```python
from build123d import *

# Parameters (mm, degrees)
SKETCH1_W          = 82.5
SKETCH1_H          = 56
MAINSHAPE_DEPTH    = 4.5
SKETCH2_W          = 10
SKETCH2_H          = 9
TAB1_DEPTH         = 4.5
CUT_EXTRUDE2_DEPTH = 53.707328712
SKETCH5_R          = 1.6
SKETCH5_W          = 4.7
SKETCH5_H          = 10.2
CUT_EXTRUDE3_DEPTH = 53.707328712
SKETCH6_R          = 11.5
CUT_EXTRUDE4_DEPTH = 53.707328712
SKETCH8_R          = 1.6
CUT_EXTRUDE6_DEPTH = 53.707328712
CUT_EXTRUDE7_DEPTH = 53.707328712


with BuildPart() as part:
    # Sketch1 → MainShape (new body)
    with BuildSketch(Plane(origin=(0, 0, 0), x_dir=(1, 0, 0), z_dir=(0, 1, 0))):
        Rectangle(SKETCH1_W, SKETCH1_H)
    extrude(amount=MAINSHAPE_DEPTH)

    # Sketch2 → Tab1 (add, through all)
    with BuildSketch(Plane(origin=(0, 4.5, 0), x_dir=(1, 0, 0), z_dir=(0, 1, 0))):
        with Locations((0, 28)):
            Rectangle(SKETCH2_W, SKETCH2_H)
    extrude(amount=-TAB1_DEPTH)

    # Sketch4 → Cut-Extrude2 (cut, through all)
    with BuildSketch(Plane(origin=(0, 4.5, 0), x_dir=(1, 0, 0), z_dir=(0, 1, 0))):
        with BuildLine():
            Line((-28.25, 17.5), (-31.75, 17.5))
            Line((-31.75, 17.5), (-31.75, 20))
            Line((-31.75, 20), (-32.75, 20))
            ThreePointArc((-32.75, 20), (-32.926776695, 20.073223305), (-33, 20.25))
            Line((-33, 20.25), (-33, 23.95))
            ThreePointArc((-33, 23.95), (-32.926776695, 24.126776695), (-32.75, 24.2))
            Line((-32.75, 24.2), (-31.75, 24.2))
            Line((-31.75, 24.2), (-31.75, 28))
            Line((-31.75, 28), (-28.25, 28))
            Line((-28.25, 28), (-28.25, 24.2))
            Line((-28.25, 24.2), (-27.25, 24.2))
            ThreePointArc((-27.25, 24.2), (-27.073223305, 24.126776695), (-27, 23.95))
            Line((-27, 23.95), (-27, 20.25))
            ThreePointArc((-27, 20.25), (-27.073223305, 20.073223305), (-27.25, 20))
            Line((-27.25, 20), (-28.25, 20))
            Line((-28.25, 20), (-28.25, 17.5))
        make_face()
        with BuildLine():
            Line((28.25, 17.5), (28.25, 20))
            Line((28.25, 20), (27.25, 20))
            ThreePointArc((27.25, 20), (27.073223305, 20.073223305), (27, 20.25))
            Line((27, 20.25), (27, 23.95))
            ThreePointArc((27, 23.95), (27.073223305, 24.126776695), (27.25, 24.2))
            Line((27.25, 24.2), (28.25, 24.2))
            Line((28.25, 24.2), (28.25, 28))
            Line((28.25, 28), (31.75, 28))
            Line((31.75, 28), (31.75, 24.2))
            Line((31.75, 24.2), (32.75, 24.2))
            ThreePointArc((32.75, 24.2), (32.926776695, 24.126776695), (33, 23.95))
            Line((33, 23.95), (33, 20.25))
            ThreePointArc((33, 20.25), (32.926776695, 20.073223305), (32.75, 20))
            Line((32.75, 20), (31.75, 20))
            Line((31.75, 20), (31.75, 17.5))
            Line((31.75, 17.5), (28.25, 17.5))
        make_face()
    extrude(amount=-CUT_EXTRUDE2_DEPTH, mode=Mode.SUBTRACT)

    # Sketch5 → Cut-Extrude3 (cut, through all)
    with BuildSketch(Plane(origin=(0, 4.5, 0), x_dir=(1, 0, 0), z_dir=(0, 1, 0))):
        with Locations(Location((34.5, -4.5, 0), (0, 0, 270))):
            Circle(SKETCH5_R)
        with Locations(Location((-34.5, -4.5, 0), (0, 0, 90))):
            Circle(SKETCH5_R)
        with Locations((34.5, 8)):
            Rectangle(SKETCH5_W, SKETCH5_H)
        with Locations((-34.5, 8)):
            Rectangle(SKETCH5_W, SKETCH5_H)
        with Locations((-34.5, -17)):
            Rectangle(SKETCH5_W, SKETCH5_H)
        with Locations((34.5, -17)):
            Rectangle(SKETCH5_W, SKETCH5_H)
    extrude(amount=-CUT_EXTRUDE3_DEPTH, mode=Mode.SUBTRACT)

    # Sketch6 → Cut-Extrude4 (cut, through all)
    with BuildSketch(Plane(origin=(0, 4.5, 0), x_dir=(1, 0, 0), z_dir=(0, 1, 0))):
        with Locations(Location((-13, 2, 0), (0, 0, 270))):
            Circle(SKETCH6_R)
    cut_extrude4 = extrude(amount=-CUT_EXTRUDE4_DEPTH, mode=Mode.SUBTRACT)

    # Sketch8 → Cut-Extrude6 (cut, through all)
    with BuildSketch(Plane(origin=(0, 4.5, 0), x_dir=(1, 0, 0), z_dir=(0, 1, 0))):
        with Locations(Location((-21, -19.46, 0), (0, 0, 270))):
            Circle(SKETCH8_R)
        with Locations(Location((-5, -19.46, 0), (0, 0, 90))):
            Circle(SKETCH8_R)
    cut_extrude6 = extrude(amount=-CUT_EXTRUDE6_DEPTH, mode=Mode.SUBTRACT)

    # Sketch9 → Cut-Extrude7 (cut, through all)
    with BuildSketch(Plane(origin=(0, 4.5, 0), x_dir=(1, 0, 0), z_dir=(0, 1, 0))):
        with BuildLine():
            Line((17.75, -28), (17.75, -24.2))
            Line((17.75, -24.2), (18.75, -24.2))
            ThreePointArc((18.75, -24.2), (18.926776695, -24.126776695), (19, -23.95))
            Line((19, -23.95), (19, -20.25))
            ThreePointArc((19, -20.25), (18.926776695, -20.073223305), (18.75, -20))
            Line((18.75, -20), (17.75, -20))
            Line((17.75, -20), (17.75, -17.5))
            Line((17.75, -17.5), (14.25, -17.5))
            Line((14.25, -17.5), (14.25, -20))
            Line((14.25, -20), (13.25, -20))
            ThreePointArc((13.25, -20), (13.073223305, -20.073223305), (13, -20.25))
            Line((13, -20.25), (13, -23.95))
            ThreePointArc((13, -23.95), (13.073223305, -24.126776695), (13.25, -24.2))
            Line((13.25, -24.2), (14.25, -24.2))
            Line((14.25, -24.2), (14.25, -28))
            Line((14.25, -28), (17.75, -28))
        make_face()
        with BuildLine():
            Line((-14.25, -28), (-14.25, -24.2))
            Line((-14.25, -24.2), (-13.25, -24.2))
            ThreePointArc((-13.25, -24.2), (-13.073223305, -24.126776695), (-13, -23.95))
            Line((-13, -23.95), (-13, -20.25))
            ThreePointArc((-13, -20.25), (-13.073223305, -20.073223305), (-13.25, -20))
            Line((-13.25, -20), (-14.25, -20))
            Line((-14.25, -20), (-14.25, -17.5))
            Line((-14.25, -17.5), (-17.75, -17.5))
            Line((-17.75, -17.5), (-17.75, -20))
            Line((-17.75, -20), (-18.75, -20))
            ThreePointArc((-18.75, -20), (-18.926776695, -20.073223305), (-19, -20.25))
            Line((-19, -20.25), (-19, -23.95))
            ThreePointArc((-19, -23.95), (-18.926776695, -24.126776695), (-18.75, -24.2))
            Line((-18.75, -24.2), (-17.75, -24.2))
            Line((-17.75, -24.2), (-17.75, -28))
            Line((-17.75, -28), (-14.25, -28))
        make_face()
    extrude(amount=-CUT_EXTRUDE7_DEPTH, mode=Mode.SUBTRACT)

    # Mirror1: Cut-Extrude4, Cut-Extrude6 across plane
    add(cut_extrude4.mirror(Plane(origin=(0, 0, 0), x_dir=(0, 0, 1), z_dir=(1, 0, 0))), mode=Mode.SUBTRACT)
    add(cut_extrude6.mirror(Plane(origin=(0, 0, 0), x_dir=(0, 0, 1), z_dir=(1, 0, 0))), mode=Mode.SUBTRACT)


solid = part.part
```
The listing builds one solid part. Answer for the finished solid, in the listing's coordinates (mm). A direction names the side the tool comes from. Round coordinates to 2 decimals unless told otherwise and drop trailing zeros. Loops run counter-clockwise (first coordinate to the right, second up) from the corner with the lowest first, then second, coordinate; pieces in that order, holes last.
Q1. Section A-A, the plane x = 34.5 is taken. Determine the outline of the cut face in (y, z), then the cut area to 3 significant figures.
Q2. Which of the six approach directions +Z, -Z, +X, -X, +Y, -Y give full straight-line access (tool end or side, diameter ignored) to faces 4 (the face through (-17.75, 2, 19)), 5 (the face through (16, 2, -28)), 6 (the face through (-35, 2, -13.1)), 7 (the face through (31.75, 2, -26))?
Q3. Section C-C, the plane z = 4.5 is taken. Determine the outline of the cut face in (x, y).
Q4. For a pull along Z with two mould halves and no side action, classify faces 1 (the face through (16, 2, 17.5)), 2 (the face through (34, 2, -13.1)), 3 (the face through (0, 2, -32.5)) as released by +Z, released by -Z, zero draft, split by the parting line, or undercut.
Q5. Find the intervals of material crossed by line 1 (X direction, y = 4, z = -26.5); line 2 (X direction, y = 2.25, z = 24.5); line 3 (X direction, y = 1.1, z = 4.5), in increasing order.
Q6. Section D-D, the plane y = 0.95 is taken. Count the separate pieces of the cut face and the enclosed holes in it, then the cut area to 3 significant figures.
Q7. Given pin 1 Ø0.8 at (x, y) = (-13.5, 2.5) entering from -Z, flat-ended and moving along its own axis, determine where the tip first touches the part or whether it passes through.
Q8. Section B-B, the plane x = -21 is taken. Determine the outline of the cut face in (y, z).
Completed:
1. outline: (0, -28) - (4.5, -28) - (4.5, -13.1) - (0, -13.1) - close; (0, -2.9) - (4.5, -2.9) - (4.5, 2.9) - (0, 2.9) - close; (0, 6.1) - (4.5, 6.1) - (4.5, 11.9) - (0, 11.9) - close; (0, 22.1) - (4.5, 22.1) - (4.5, 28) - (0, 28) - close
1. area: 146 mm2
2. face 4: +Z, +Y, -Y
2. face 5: -Z, +X, +Y, -Y
2. face 6: +Y, -Y
2. face 7: -Z, +Y, -Y
3. outline: (-41.25, 0) - (-36.1, 0) - (-36.1, 4.5) - (-41.25, 4.5) - close; (-32.9, 0) - (-22.49, 0) - (-22.49, 4.5) - (-32.9, 4.5) - close; (-3.51, 0) - (3.51, 0) - (3.51, 4.5) - (-3.51, 4.5) - close; (22.49, 0) - (32.9, 0) - (32.9, 4.5) - (22.49, 4.5) - close; (36.1, 0) - (41.25, 0) - (41.25, 4.5) - (36.1, 4.5) - close
4. face 1: released by +Z
4. face 2: undercut
4. face 3: released by -Z
5. line 1: x = -41.25 to -31.75, -28.25 to 28.25, 31.75 to 41.25
5. line 2: x = -41.25 to -17.75, -14.25 to 14.25, 17.75 to 41.25
5. line 3: x = -41.25 to -36.1, -32.9 to -22.49, -3.51 to 3.51, 22.49 to 32.9, 36.1 to 41.25
6. separate pieces: 1
6. enclosed holes: 12
6. area: 3,410 mm2
7. pin 1: stops at z = -28
8. outline: (0, -28) - (4.5, -28) - (4.5, -10.26) - (0, -10.26) - close; (0, 6.26) - (4.5, 6.26) - (4.5, 17.86) - (0, 17.86) - close; (0, 21.06) - (4.5, 21.06) - (4.5, 28) - (0, 28) - close
